Print and shaded views of the part. All mm, measured from the part's lowest x, y and z. Give positions to 0.01 mm unless a question says otherwise; leave off trailing zeros. Loops run counter-clockwise (first coordinate to the right, second up) from the corner with the lowest first, then second, coordinate; pieces in that order, holes last. Notation, with made-up numbers: (20, 19) - (68, 19) arc R13 ccw to (68, 41) - close; hole circle Ø7 at (10, 76). An arc over 180 degrees is marked (long way). Return JSON: item names as keys, results as strings.
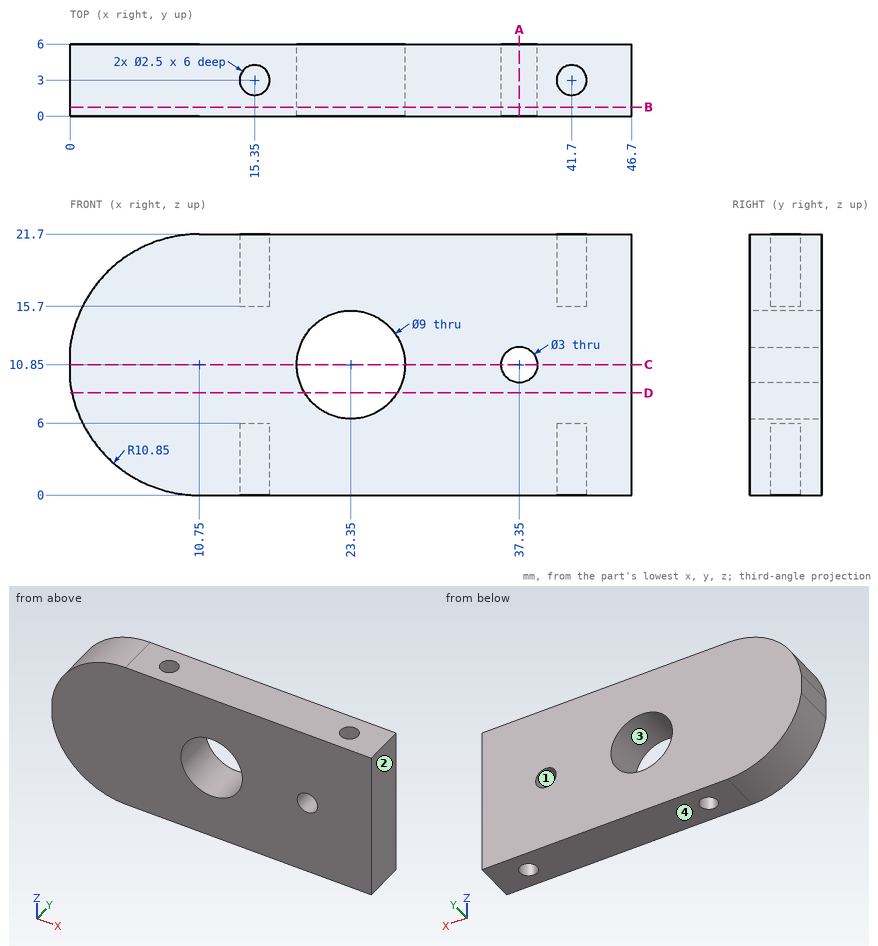
1. Pull direction X, two halves, no side cores. Call the marked faces 1, 2, 3 and 4: +X half, -X half, draft (parallel to the pull), parting line (faces both ways), or undercut.
Values follow:
{"face 1": "undercut", "face 2": "+X half", "face 3": "undercut", "face 4": "draft"}
2. Cut at A-A, the plane x = 37.35. Write the cut outline in (y, z).
Values follow:
{"outline": "(0, 0) - (6, 0) - (6, 9.35) - (0, 9.35) - close; (0, 12.35) - (6, 12.35) - (6, 21.7) - (0, 21.7) - close"}
3. Cut at D-D, the plane z = 8.5. Write the cut outline in (x, y), plus the area to 3 significant figures.
Values follow:
{"outline": "(0.16, 0) - (19.51, 0) - (19.51, 6) - (0.16, 6) - close; (27.19, 0) - (46.7, 0) - (46.7, 6) - (27.19, 6) - close", "area": "233 mm²"}
4. Drill centre lines: probe 1 along X at (y, z) = (5.1, 10.75); probe 2 along Y at (x, z) = (15.35, 19.5); probe 3 along Z at (x, y) = (37, 5.75). Where is each one in solid material? Low to high.
Values follow:
{"probe 1": "x = 0 to 18.85, 27.85 to 35.85, 38.85 to 46.7", "probe 2": "y = 0 to 1.75, 4.25 to 6", "probe 3": "z = 0 to 9.39, 12.31 to 21.7"}
5. Drop flat-ended pins along their axis: P1, Ø1.5, axis at x = 15.35, y = 3, coming from the -Z side; P2, Ø2, axis at y = 1, z = 7, coming from the -X side. Give the stop position or say it passes through.
Values follow:
{"P1": "stops at z = 6", "P2": "stops at x = 0.28"}
6. Cut at C-C, the plane z = 10.85. Write the cut outline in (x, y).
Values follow:
{"outline": "(0, 0) - (18.85, 0) - (18.85, 6) - (0, 6) - close; (27.85, 0) - (35.85, 0) - (35.85, 6) - (27.85, 6) - close; (38.85, 0) - (46.7, 0) - (46.7, 6) - (38.85, 6) - close"}
7. Cut at B-B, the plane y = 0.75. Write the cut outline in (x, z), plus the area to 3 significant figures.
Values follow:
{"outline": "(0, 9.38) arc R10.85 ccw to (10.75, 0) - (46.7, 0) - (46.7, 21.7) - (10.75, 21.7) arc R10.85 ccw to (0, 12.32) - close; hole circle Ø9 at (23.35, 10.85); hole circle Ø3 at (37.35, 10.85)", "area": "894 mm²"}
